Can you work these out from the model? Positions are in its coordinate system, mm. Give positions to 0.01 mm unless a question says otherwise; leave off trailing zeros. Loops run counter-clockwise (first coordinate to the right, second up) from the corner with the lowest first, then second, coordinate; pieces in that order, holes last. Notation, with made-up numbers: M 34,-11 L 76,-11 A5 ccw 76,-5 Z; hole C 40.5,-37 d11. An arc over 180 degrees is marked long. Put each result on its own line as item: value. Start each with the question number.
1) Please list where these lines run through material, in increasing order: line 1 along Y through (x, z) = (-4, 3.1); line 2 along X through (y, z) = (10, 1.85); line 3 along Y through (x, z) = (0, 2.7). Write a range as from..to.
2) Imagine slicing it at D-D (z = 2.2). Write out the boundary of the cut face in (x, y).
3) Imagine slicing it at B-B (x = -2). Write out the boundary of the cut face in (y, z).
4) Imagine slicing it at C-C (x = 0). Write out the boundary of the cut face in (y, z), then the cut area to 3 significant figures.
5) Imagine slicing it at A-A (y = 10). Write out the boundary of the cut face in (x, z), then the cut area to 3 significant figures.
6) If we mould it in two halves opening along X, with no side actions, what happens to faces 1 (the flat face through (0, 15, 2)), 2 (the flat face through (-10, 0, 2)), 3 (the cylindrical face through (-1, 10, 2)), 4 (the cylindrical face through (0.65, -2.07, 2.03))? For each: +X half, -X half, draft (parallel to the pull), parting line (faces both ways), or undercut.
from build123d import *

# Parameters (mm, degrees)
F1_DEPTH = 4
F2_D     = 6
F3_D     = 6


with BuildPart() as f1:
    # F0 (on Top) → F1 (new body)
    with BuildSketch(Plane.XY):
        Polygon((10, 15), (-10, 15), (-10, -15), (0, -15), (10, -15), align=None)
    extrude(amount=F1_DEPTH)

    # F2 (through all)
    with Locations(Plane(origin=(0, 0, 0), x_dir=(1, 0, 0), z_dir=(0, 0, -1))):
        with Locations((-4, -10)):
            Hole(F2_D / 2)

    # F3 (through all)
    with Locations(Plane(origin=(0, 0, 0), x_dir=(1, 0, 0), z_dir=(0, 0, -1))):
        with Locations((0, 5)):
            Hole(F3_D / 2)


solid = f1.part
Recorded:
1. line 1: -15..7, 13..15
1. line 2: -10..-7, -1..10
1. line 3: -15..-8, -2..15
2. outline: M -10,-15 L 10,-15 L 10,15 L -10,15 Z; hole C -4,10 d6; hole C 0,-5 d6
3. outline: M -15,0 L -7.24,0 L -7.24,4 L -15,4 Z; M -2.76,0 L 7.76,0 L 7.76,4 L -2.76,4 Z; M 12.24,0 L 15,0 L 15,4 L 12.24,4 Z
4. outline: M -15,0 L -8,0 L -8,4 L -15,4 Z; M -2,0 L 15,0 L 15,4 L -2,4 Z
4. area: 96.0 mm²
5. outline: M -10,0 L -7,0 L -7,4 L -10,4 Z; M -1,0 L 10,0 L 10,4 L -1,4 Z
5. area: 56.0 mm²
6. face 1: draft
6. face 2: -X half
6. face 3: undercut
6. face 4: undercut
